Here's the drawing with two shaded views (mm, measured from the low corner). I have some questions. Coordinates: 2 decimals unless noted, no trailing zeros. Write each loop counter-clockwise with the first axis right and the second up, starting at its lowest first coordinate (ties: lowest second). Pieces come first, ordered by that corner, then holes.
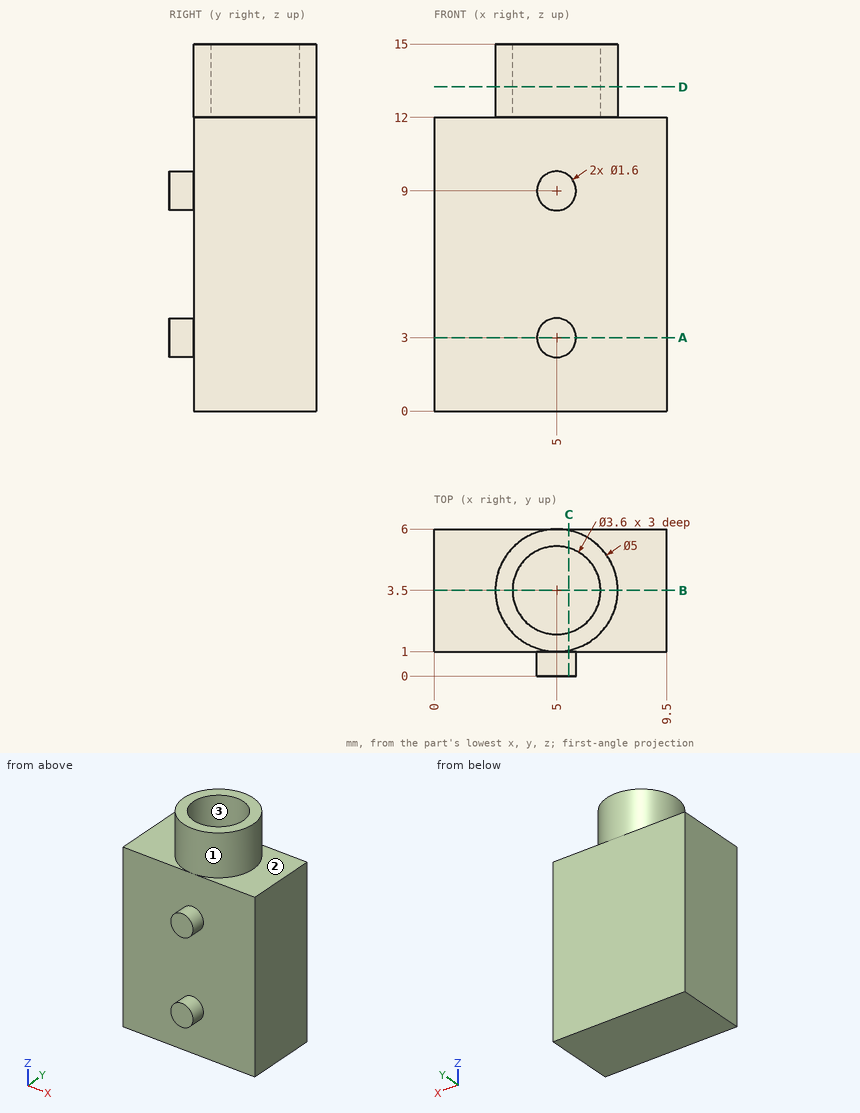
1. Please list where these lines run through material, in increasing order: line 1 along Y through (x, z) = (5, 13.8); line 2 along Y through (x, z) = (8.75, 6.5); line 3 along Z through (x, y) = (6.5, 2.9).
Verdict:
line 1: y = 1 to 1.7, 5.3 to 6
line 2: y = 1 to 6
line 3: z = 0 to 12
2. I want a section at C-C on x = 5.5. Please give me the cut outline in (y, z), plus the area to 3 significant figures.
Verdict:
outline: (0, 2.38) - (1, 2.38) - (1, 0) - (6, 0) - (6, 12) - (5.95, 12) - (5.95, 15) - (5.23, 15) - (5.23, 12) - (1.77, 12) - (1.77, 15) - (1.05, 15) - (1.05, 12) - (1, 12) - (1, 9.62) - (0, 9.62) - (0, 8.38) - (1, 8.38) - (1, 3.62) - (0, 3.62) - close
area: 66.8 mm2
3. If we mould it in two halves opening along X, with no side actions, what happens to the marked faces 1, 2 and 3? For each: pulls with the +X half, pulls with the -X half, needs draft (parallel to the pull), parting line crosses it, or undercut.
Verdict:
face 1: parting line crosses it
face 2: needs draft
face 3: undercut
4. I want a section at A-A on z = 3. Please give me the cut outline in (x, y), plus the area to 3 significant figures.
Verdict:
outline: (0, 1) - (4.2, 1) - (4.2, 0) - (5.8, 0) - (5.8, 1) - (9.5, 1) - (9.5, 6) - (0, 6) - close
area: 49.1 mm2
5. I want a section at D-D on z = 13.25. Please give me the cut outline in (x, y).
Verdict:
outline: circle Ø5 at (5, 3.5); hole circle Ø3.6 at (5, 3.5)
6. For pin 1 (1.1 mm diameter, centred on x = 4.5, y = 4.5, fed in from +Z), with a flat end and sliding along its axis, tell me the tip position at first contact or that it passes through.
Verdict:
pin 1: stops at z = 12
7. I want a section at B-B on y = 3.5. Please give me the cut outline in (x, z), plus the area to 3 significant figures.
Verdict:
outline: (0, 0) - (9.5, 0) - (9.5, 12) - (7.5, 12) - (7.5, 15) - (6.8, 15) - (6.8, 12) - (3.2, 12) - (3.2, 15) - (2.5, 15) - (2.5, 12) - (0, 12) - close
area: 118 mm2
